Check sheet for the modelled part. Datum: model origin and axes. Units: mm. Face numbers are marked on the shaded views. A direction names the side the tool comes from. Give positions to 0.01 mm unless a question says otherwise; leave off trailing zeros. Order: outer loops, then holes, each group sorted by start corner. A loop starts at its lowest first (then second) coordinate and runs counter-clockwise, first axis right, second up. Notation, with made-up numbers: M 32.5,65 L 73.5,65 A38 ccw 73.5,104 Z; hole C -5,-1.5 d6. An arc over 180 degrees is marked long. Answer in a Markdown table with one row per item. Add a question column.
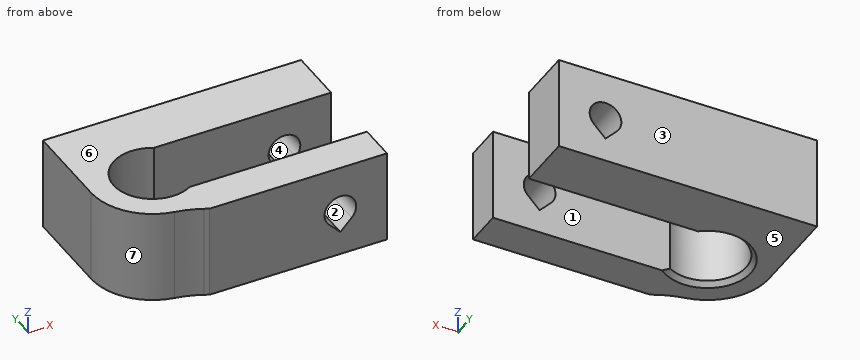
Solid Edge part; units mm, degrees
sketch "Sketch1" plane through (0, 0, 0) normal (0, 0, 1) x (1, 0, 0)
  line L0 (2.075, 3.594) -> (21.075, 3.594)
  line L1 (21.075, 9.594) -> (21.075, 3.594)
  line L2 (21.075, 9.594) -> (-7.594, 9.594)
  line L3 (-7.594, 0) -> (-7.594, 9.594)
  line L4 (21.075, -7.594) -> (0, -7.594)
  line L5 (21.075, -7.594) -> (21.075, -3.594)
  line L6 (2.075, -3.594) -> (21.075, -3.594)
  arc A0 (2.075, -3.594) -> (2.075, 3.594) centre (0, 0) cw
  arc A1 (-7.594, 0) -> (0, -7.594) centre (0, 0) ccw
extrude "Protrusion1" add sketch "Sketch1" along normal blind 10
sketch "Sketch2" plane through (-2.2595, 7.594, 5) normal (0, 1, 0) x (1, 0, 0)
  line L0 (19.5574, 1.1809) -> (18.3345, 2.4472)
  line L1 (18.3345, 2.4472) -> (17.1116, 1.1809)
  arc A0 (19.5574, 1.1809) -> (17.1116, 1.1809) centre (18.3345, 0) cw
extrude "Cutout1" cut sketch "Sketch2" along normal through all and the other way through all
sketch "Sketch3" plane through (6.7405, 1, 10) normal (0, 0, 1) x (1, 0, 0)
  line L0 (-14.3345, 8.594) -> (-13.3345, 8.594)
  line L1 (-13.3345, 8.594) -> (-13.3345, -1)
  arc A0 (-13.3345, -1) -> (-7.8394, -7.5018) centre (-6.7405, -1) ccw
  arc A1 (-5.1645, -8.3535) -> (-7.8394, -7.5018) centre (-9.506, -17.3619) ccw
  line L2 (-5.1645, -8.3535) -> (-4.6655, -8.594)
  dimension "D1" = 14.3345
extrude "Cutout2" cut sketch "Sketch3" against normal through all material side at (-7.094, 9.544, 10)
chamfer "Chamfer_2" distance 0.5 angle 45 1 edges at (-4.15, 0, 0)
properties material "ABS Plastic, medium impact"
Q1. Thickness scan on probe 1 along Y at (x, z) = (8, 6.5); probe 2 along X at (y, z) = (6.35, 5) (3 decimals); probe 3 along Y at (x, z) = (-1.25, 3). Record the ranges inside material, lowest first.
Q2. Draft check along Z on the marked faces 4, 5, 6 and 7. Enter one of: pulls with the +Z half, pulls with the -Z half, needs draft (parallel to the pull), parting line crosses it, or undercut.
Q3. Cross-section at B-B (y = 5.25). Record the boundary of the cut face in (x, z) (3 decimals).
Q4. Cross-section at C-C (z = 5). State how many separate pieces and enclosed holes the cut face has, and give its area (3 significant figures).
Q5. Cross-section at A-A (x = 5.25). Record the boundary of the cut face in (y, z), and give its area (4 significant figures).
Q6. Tool access check on the marked faces 1, 2 and 3. Record the directions out of +Z, -Z, +X, -X, +Y, -Y that give a thin tool (end or side, any length) a straight path to the whole face; none if there is none.
Q7. Go/stop test with a flat-tipped pin: pin 1 (2 mm diameter, centred on x = 16.075, z = 5, fed in from -Y). Record where the tip stops, or that it passes through.
Values follow:
| question | item | result |
|---|---|---|
| 1 | probe 1 | -7.59 to -3.59, 3.59 to 9.59 |
| 1 | probe 2 | -6.594 to 14.375, 17.775 to 21.075 |
| 1 | probe 3 | -6.47 to -3.96, 3.96 to 9.59 |
| 2 | face 4 | undercut |
| 2 | face 5 | pulls with the -Z half |
| 2 | face 6 | pulls with the +Z half |
| 2 | face 7 | needs draft |
| 3 | outline | M -6.594,0 L 21.075,0 L 21.075,10 L -6.594,10 Z; hole M 14.852,3.819 L 16.075,2.553 L 17.298,3.819 A1.7 ccw long Z |
| 4 | separate pieces | 3 |
| 4 | enclosed holes | 0 |
| 4 | area | 245 mm² |
| 5 | outline | M -7.59,0 L -3.59,0 L -3.59,10 L -7.59,10 Z; M 3.59,0 L 9.59,0 L 9.59,10 L 3.59,10 Z |
| 5 | area | 100.0 mm² |
| 6 | face 1 | +Z, -Z, +X |
| 6 | face 2 | +Y, -Y |
| 6 | face 3 | +Z, -Z, +X, -X, +Y |
| 7 | pin 1 | through |
